```python
from build123d import *

# Parameters (mm, degrees)
F1_R     = 4
F2_DEPTH = 10
F3_R     = 20
F4_R     = 40


with BuildPart() as f2:
    # F1 (on Right) → F2 (new body)
    with BuildSketch(Plane.YZ):
        Polygon((-284.6176624298, -40), (-145, -40), (0, -40), (145, -40), (284.6176624298, -40), (243.3743673133, 33.5336461051), (28.7415579511, 405.2885768915), (0, 425.2763390541), (-28.7415579511, 405.2885768915), (-243.3743673133, 33.5336461051), align=None)
        with Locations((-202.9333580064, -26.6499444856)):
            Circle(F1_R, mode=Mode.SUBTRACT)
        with Locations((-231.9333580064, 23.5795289339)):
            Circle(F1_R, mode=Mode.SUBTRACT)
        with Locations((-29, -20)):
            Circle(F1_R, mode=Mode.SUBTRACT)
        with Locations((29, -20)):
            Circle(F1_R, mode=Mode.SUBTRACT)
        with Locations((202.9333580064, -26.6499444856)):
            Circle(F1_R, mode=Mode.SUBTRACT)
        with Locations((231.9333580064, 23.5795289339)):
            Circle(F1_R, mode=Mode.SUBTRACT)
        with BuildLine():
            Line((205, 0), (0, 0))
            Line((0, 0), (-205, 0))
            Line((-205, 0), (-200.0730971241, 8.5336461051))
            Line((-200.0730971241, 8.5336461051), (-40, 285.7883832489))
            ThreePointArc((-40, 285.7883832489), (-40, 331.976404784), (0, 355.0704155516))
            ThreePointArc((0, 355.0704155516), (40, 331.976404784), (40, 285.7883832489))
            Line((40, 285.7883832489), (200.0730971241, 8.5336461051))
            Line((200.0730971241, 8.5336461051), (205, 0))
        make_face(mode=Mode.SUBTRACT)
        with Locations((-29, 375.0704155516)):
            Circle(F1_R, mode=Mode.SUBTRACT)
        with Locations((29, 375.0704155516)):
            Circle(F1_R, mode=Mode.SUBTRACT)
    extrude(amount=F2_DEPTH)

    # F3
    f3_edges = [f2.edges().sort_by_distance(p)[0] for p in [
        (5, -284.617662, -40),
        (5, 284.617662, -40),
        (5, 0, 425.276339),
        (5, -40, 285.788383),
        (5, 40, 285.788383),
    ]]
    fillet(f3_edges, radius=F3_R)

    # F4
    f4_edges = [f2.edges().sort_by_distance(p)[0] for p in [
        (5, 205, 0),
        (5, -205, 0),
    ]]
    fillet(f4_edges, radius=F4_R)


solid = f2.part
```
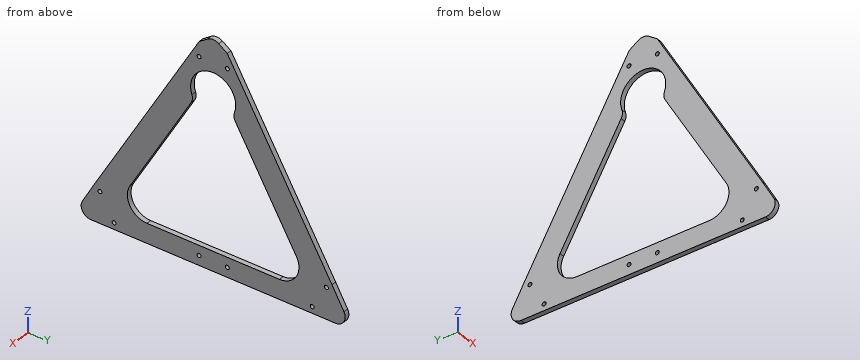
Geometry: final body of the model. Coordinates: model frame, mm. Coordinates: 2 decimals unless noted, no trailing zeros. Order: outer loops, then holes, each group sorted by start corner. A loop starts at its lowest first (then second) coordinate and runs counter-clockwise, first axis right, second up. Notation, with made-up numbers: (-23, 88.5) -> (5, 88.5) arc R22 cw to (5, 110.5) -> close; hole circle Ø1 at (16, 22). An arc over 180 degrees is marked (long way). Answer in a Markdown table with one row per item.
Item 1: Section D-D on z = 392. Output: boundary loops of the cut face in (x, y).
Return value:
| item | result |
|---|---|
| outline | (0, -36.41) -> (10, -36.41) -> (10, 36.41) -> (0, 36.41) -> close |
Item 2: Section A-A on y = 0. Output: boundary loops of the cut face in (x, z), plus the area to 3 significant figures.
Return value:
| item | result |
|---|---|
| outline | (0, -40) -> (10, -40) -> (10, 0) -> (0, 0) -> close; (0, 355.07) -> (10, 355.07) -> (10, 420.92) -> (0, 420.92) -> close |
| area | 1,060 mm² |
Item 3: Section C-C on x = 6.5. State how many separate pieces and enclosed holes the cut face has, plus the area to 3 significant figures.
Return value:
| item | result |
|---|---|
| separate pieces | 1 |
| enclosed holes | 9 |
| area | 66,300 mm² |
Item 4: Section B-B on z = 150. Output: boundary loops of the cut face in (x, y), plus the area to 3 significant figures.
Return value:
| item | result |
|---|---|
| outline | (0, -176.13) -> (10, -176.13) -> (10, -118.4) -> (0, -118.4) -> close; (0, 118.4) -> (10, 118.4) -> (10, 176.13) -> (0, 176.13) -> close |
| area | 1,150 mm² |
Item 5: Contact query for flat-ended pins moving along their axis: P1, Ø3, axis at x = 7, y = 26, coming from the +Z side; P2, Ø1, axis at x = 2.5, y = -123, coming from the +Z side; P3, Ø4, axis at x = 2.5, y = -29, coming from the +Z side. Output: stop coordinate, or through.
Return value:
| item | result |
|---|---|
| P1 | stops at z = 408.24 |
| P2 | stops at z = 242.89 |
| P3 | stops at z = 406.5 |
Item 6: Ray query, L1, parallel to Z at x = 7.5, y = 29; L2, parallel to Z at x = 0.5, y = -72.5; L3, parallel to Y at x = 7.5, z = 274.5. Return the intervals inside material, ascending.
Return value:
| item | result |
|---|---|
| L1 | z = -40 to -24, -16 to 0, 344.83 to 371.07, 379.07 to 404.84 |
| L2 | z = -40 to 0, 229.5 to 329.5 |
| L3 | y = -104.25 to -46.52, 46.52 to 104.25 |
